Source: CAD feature listing. Evaluate the final solid. Frame: model axes, mm. A direction names the side the tool comes from. Give positions to 0.01 mm unless a question says otherwise; leave off trailing zeros. Write each loop counter-clockwise with the first axis right and the second up, starting at its lowest first coordinate (ties: lowest second). Pieces come first, ordered by that corner, then holes.
```python
from build123d import *

# Parameters (mm, degrees)
BOSS_EXTRUDE1_DEPTH = 6
SKETCH2_R           = 1
SKETCH2_W           = 3
SKETCH2_H           = 3
CUT_EXTRUDE1_DEPTH  = 23.226110771
FILLET1_R           = 4


with BuildPart() as part:
    # Sketch1 → Boss-Extrude1 (new body)
    with BuildSketch(Plane(origin=(0, 0, 0), x_dir=(1, 0, 0), z_dir=(0, 1, 0))):
        Polygon((3.5, 0), (3.5, 4), (9.5, 4), (9.5, 0), (13, 0), (13, 17), (0, 17), (0, 0), align=None)
    extrude(amount=BOSS_EXTRUDE1_DEPTH)

    # Sketch2 → Cut-Extrude1 (cut, through all)
    with BuildSketch(Plane(origin=(0, 6, 0), x_dir=(1, 0, 0), z_dir=(0, 1, 0))):
        with Locations(Location((6.5, 6, 0), (0, 0, 270))):
            Circle(SKETCH2_R)
        with Locations((6.5, 11.5)):
            Rectangle(SKETCH2_W, SKETCH2_H)
    extrude(amount=-CUT_EXTRUDE1_DEPTH, mode=Mode.SUBTRACT)

    # Fillet1
    fillet1_edges = [part.edges().sort_by_distance(p)[0] for p in [
        (0, 3, -17),
        (13, 3, -17),
    ]]
    fillet(fillet1_edges, radius=FILLET1_R)


solid = part.part
```
1. Line query: probe 1 along X at (y, z) = (2.15, -3.5); probe 2 along X at (y, z) = (1.4, -6); probe 3 along Z at (x, y) = (8.5, 1.25). Output: solid intervals per line, ascending.
2. Pin query (flat end, axial travel): P1, Ø3.5, axis at x = 7, y = 3, coming from the +Z side. Return the tip coordinate at first contact, or that it passes through.
3. Section query A-A (z = -2.75). Return loops of the section in (x, y), plus the area to 3 significant figures.
4. Section query D-D (z = -10.75). Return loops of the section in (x, y), plus the area to 3 significant figures.
5. Section query C-C (y = 3.6). Return loops of the section in (x, z), plus the area to 3 significant figures.
6. Access query for faces 1 (the flat face through (7, 3, -17)), 2 (the flat face through (6, 3, -4)), 3 (the flat face through (5, 3, -11)). Directions: +Z, -Z, +X, -X, +Y, -Y. A direction counts if a zero-diameter tool reaches every point of the face in a straight line with its end or side. Return the directions, or none.
7. Section query B-B (x = 6.5). Return loops of the section in (y, z).
8. Pull-direction query (X, two-part tool) for faces 4 (the flat face through (6, 6, -9)), 5 (the flat face through (6, 3, -10)), 6 (the cylindrical face through (11.797, 3.042, -15.859)); classes: pulls with the +X half, pulls with the -X half, needs draft (parallel to the pull), parting line crosses it, or undercut.
The answers:
1. probe 1: x = 0 to 3.5, 9.5 to 13
1. probe 2: x = 0 to 5.5, 7.5 to 13
1. probe 3: z = -17 to -4
2. P1: stops at z = -4
3. outline: (0, 0) - (3.5, 0) - (3.5, 6) - (0, 6) - close; (9.5, 0) - (13, 0) - (13, 6) - (9.5, 6) - close
3. area: 42.0 mm2
4. outline: (0, 0) - (5, 0) - (5, 6) - (0, 6) - close; (8, 0) - (13, 0) - (13, 6) - (8, 6) - close
4. area: 60.0 mm2
5. outline: (0, -13) arc R4 ccw to (4, -17) - (9, -17) arc R4 ccw to (13, -13) - (13, 0) - (9.5, 0) - (9.5, -4) - (3.5, -4) - (3.5, 0) - (0, 0) - close; hole (5, -13) - (8, -13) - (8, -10) - (5, -10) - close; hole circle Ø2 at (6.5, -6)
5. area: 178 mm2
6. face 1: -Z, +X, -X, +Y, -Y
6. face 2: +Z, +Y, -Y
6. face 3: +Y, -Y
7. outline: (0, -17) - (6, -17) - (6, -13) - (0, -13) - close; (0, -10) - (6, -10) - (6, -7) - (0, -7) - close; (0, -5) - (6, -5) - (6, -4) - (0, -4) - close
8. face 4: needs draft
8. face 5: undercut
8. face 6: pulls with the +X half
